Autodesk Inventor part; units mm, degrees
ref_plane "YZ Plane" through (0, 0, 0) normal (1, 0, 0) x (0, 1, 0)
ref_plane "XZ Plane" through (0, 0, 0) normal (0, 1, 0) x (-1, 0, 0)
ref_plane "XY Plane" through (0, 0, 0) normal (0, 0, 1) x (1, 0, 0)
sketch "Sketch1" plane through (0, 0, 0) normal (0, 0, 1) x (1, 0, 0)
  circle A0 centre (0, 0) radius 20
  dimension "d0" = 40
extrude "Extrusion1" add sketch "Sketch1" along normal blind 6.6
sketch "Sketch3" plane through (0, 0, 0) normal (0, 0, -1) x (-1, 0, 0)
  circle A0 centre (0, 0) radius 17
  line L0 (0, 17) -> (0, 0)
  line L1 (0, 0) -> (14.7224, -8.5)
  line L2 (0, 0) -> (-14.7224, -8.5)
  line L3 (0, 0) -> (17, 0) construction
  line L4 (1.5, 16.9337) -> (1.5, 0.866)
  line L5 (-1.5, 16.9337) -> (-1.5, 0.866)
  line L6 (-1.5, 0.866) -> (-15.415, -7.1678)
  line L7 (0, -1.7321) -> (-13.915, -9.7659)
  line L8 (1.5, 0.866) -> (15.415, -7.1678)
  line L9 (0, -1.7321) -> (13.915, -9.7659)
  dimension "d6" = 34
  dimension "d7" = 120
  dimension "d8" = 150
  dimension "d9" = 1.5
  dimension "d10" = 1.5
  dimension "d11" = 1.5
  dimension "d12" = 1.5
  dimension "d13" = 1.5
  dimension "d14" = 1.5
extrude "Extrusion3" cut sketch "Sketch3" against normal up to surface (6.6 mm away) contours A0 L8 L4 | L5 L6 A0 | A0 L7 L9
sketch "Sketch5" plane through (0, 0, 6.6) normal (0, 0, 1) x (1, 0, 0)
  circle A0 centre (0, 0) radius 4
  dimension "d20" = 8
extrude "Extrusion5" add sketch "Sketch5" against normal blind 6.6
sketch "Sketch6" plane through (0, 0, 0) normal (0, 0, -1) x (-1, 0, 0)
  circle A0 centre (0, 0) radius 1.75
  line L0 (0, -1.75) -> (0, -4)
  arc A1 (-2.4613, -3.1531) -> (2.4613, -3.1531) centre (0, 0) ccw
  line L1 (0.5, -1.6771) -> (0.5, -3.9686)
  line L2 (-0.5, -1.6771) -> (-0.5, -3.9686)
  line L3 (-1.4697, 0.95) -> (1.4697, 0.95)
  point P0 (0.0845, 0.95)
  dimension "d23" = 3.5
  dimension "d24" = 0.5
  dimension "d25" = 0.5
  dimension "d29" = 2.7
extrude "Extrusion6" cut sketch "Sketch6" against normal up to surface (6.6 mm away) contours A0 L3 | L1 A1 L0 A0 | L0 A1 L2 A0 picked at (-0.299, -0.0924)
fillet "Arredondamento1" radius 1 2 edges at (-20, 0, 6.6) (-20, 0, 0)
properties part number "wheel35mmV1"
Part model, mm, in its own coordinate system. A direction names the side the tool comes from. Round coordinates to 2 decimals unless told otherwise and drop trailing zeros. Loops run counter-clockwise (first coordinate to the right, second up) from the corner with the lowest first, then second, coordinate; pieces in that order, holes last. Notation, with made-up numbers: (83, 0) -> (142, 0) arc R31 cw to (142, 25) -> close; hole circle Ø3 at (40, 52.5). An arc over 180 degrees is marked (long way). Use one line per item in the form item = value. Start each with the question number.
Item 1: Band-saw the part on C-C (z = 4.75). List the corners of the cut face in (x, y) (3 decimals).
Item 2: Band-saw the part on D-D (x = 8.5). Give the number of separate pieces and of enclosed holes in the cut face, plus the area to 3 significant figures.
Item 3: Drill centre lines: line 1 along Y through (x, z) = (2.5, 3.5); line 2 along X through (y, z) = (10.5, 5.25); line 3 along X through (y, z) = (12.5, 5.75). Where is each one in solid material? Low to high.
Item 4: Tool access for faces 1 (the flat face through (0.5, -3, 3)), 2 (the flat face through (0, 3, 6.6)): list every direction of +Z, -Z, +X, -X, +Y, -Y with a clear straight run to the whole face (end or side of a thin tool).
Item 5: Band-saw the part on A-A (y = 0). List the corners of the cut face in (x, z), plus the area to 3 significant figures.
Item 6: Drop flat-ended pins along their axis: pin 1 Ø2.5 at (y, z) = (-3, 2.5) entering from +X; pin 2 Ø1 at (x, z) = (-15.5, 6) entering from +Y; pin 3 Ø3.5 at (y, z) = (10.5, 4.5) entering from -X. Give the stop position or say it passes through.
Item 7: Two-plate mould, pull along Y, no slides. Class faces 3 (the cylindrical face through (-4.336, 19.524, 3.268)), 4 (the flat face through (9.608, -3.815, 3.254)), 5 (the flat face through (0, 3, 0)): released by +Y, released by -Y, zero draft, split by the parting line, or undercut.
Item 8: Band-saw the part on B-B (x = 0). List the corners of the cut face in (y, z), plus the area to 3 significant figures.
Data:
q1.outline = circle Ø40 at (0, 0); hole (-15.415, -7.168) -> (-3.961, -0.555) arc R4 cw to (-1.5, 3.708) -> (-1.5, 16.934) arc R17 ccw to start; hole (-13.915, -9.766) arc R17 ccw to (13.915, -9.766) -> (2.461, -3.153) arc R4 cw to (0.5, -3.969) -> (0.5, -1.677) arc R1.75 ccw to (1.47, 0.95) -> (-1.47, 0.95) arc R1.75 ccw to (-0.5, -1.677) -> (-0.5, -3.969) arc R4 cw to (-2.461, -3.153) -> close; hole (1.5, 3.708) arc R4 cw to (3.961, -0.555) -> (15.415, -7.168) arc R17 ccw to (1.5, 16.934) -> close
q2.separate_pieces = 3
q2.enclosed_holes = 0
q2.area = 66.5 mm^2
q3.line_1 = -19.84 to -16.82, -3.18 to 3.12, 16.82 to 19.84
q3.line_2 = -17.02 to -13.37, -1.5 to 1.5, 13.37 to 17.02
q3.line_3 = -15.6 to -11.52, -1.5 to 1.5, 11.52 to 15.6
q4.face_1 = +Z, -Z
q4.face_2 = +Z, +X, -X, +Y, -Y
q5.outline = (-20, 1) arc R1 ccw to (-19, 0) -> (-17, 0) -> (-17, 6.6) -> (-19, 6.6) arc R1 ccw to (-20, 5.6) -> close; (-4, 0) -> (-1.75, 0) -> (-1.75, 6.6) -> (-4, 6.6) -> close; (1.75, 0) -> (4, 0) -> (4, 6.6) -> (1.75, 6.6) -> close; (17, 0) -> (19, 0) arc R1 ccw to (20, 1) -> (20, 5.6) arc R1 ccw to (19, 6.6) -> (17, 6.6) -> close
q5.area = 68.4 mm^2
q6.pin_1 = 19.92
q6.pin_2 = 13.15
q6.pin_3 = -17.98
q7.face_3 = split by the parting line
q7.face_4 = undercut
q7.face_5 = zero draft
q8.outline = (-20, 1) arc R1 ccw to (-19, 0) -> (-17, 0) -> (-17, 6.6) -> (-19, 6.6) arc R1 ccw to (-20, 5.6) -> close; (0.95, 0) -> (19, 0) arc R1 ccw to (20, 1) -> (20, 5.6) arc R1 ccw to (19, 6.6) -> (0.95, 6.6) -> close
q8.area = 145 mm^2
